Can you work these out from the model? Positions are in its coordinate system, mm. Face numbers are marked on the shaded views. A direction names the side the tool comes from. Round coordinates to 2 decimals unless told otherwise and drop trailing zeros. Order: outer loops, then holes, each group sorted by start corner. A loop starts at its lowest first (then second) coordinate and runs counter-clockwise, first axis right, second up. Notation, with made-up numbers: (86.5, 86.5) - (97.5, 86.5) arc R26 ccw to (97.5, 117.5) - close; hole circle Ø4 at (-9.5, -39). An arc over 180 degrees is marked (long way). Write item = value, one per line.
from build123d import *

# Parameters (mm, degrees)
ESQUISSE1_W             = 7.9
ESQUISSE1_H             = 8.25
BOSS_EXTRU_1_DEPTH      = 1.184
ENL_V_MAT_EXTRU_1_REACH = 15.462
BOSS_EXTRU_2_DEPTH      = 1.184
ENL_V_MAT_EXTRU_2_REACH = 15.462
ESQUISSE8_R             = 7.2925
BOSS_EXTRU_3_DEPTH      = 0.296
ESQUISSE9_R             = 6.10875
BOSS_EXTRU_4_DEPTH      = 0.74
BOSS_EXTRU_4_DRAFT      = -17.000658211
ESQUISSE10_R            = 6.335
BOSS_EXTRU_5_DEPTH      = 0.444
D_POUILLE1_ANGLE        = 44.999999999
PER_AGE1_D              = 8.376
CHANFREIN1_SIZE         = 0.812
CONG_1_R                = 0.825


with BuildPart() as part:
    # Esquisse1 → Révolution1 (revolve)
    with BuildSketch(Plane.XY, mode=Mode.PRIVATE) as r_volution1_sk:
        with Locations((5.43, 4.125)):
            Rectangle(ESQUISSE1_W, ESQUISSE1_H)
    revolve(r_volution1_sk.sketch.rotate(Axis((1.48, 0, 0), (1, 0, 0)), 270), axis=Axis((1.48, 0, 0), (1, 0, 0)))

    # Esquisse2 → Boss.-Extru.1 (add)
    with BuildSketch(Plane(origin=(9.38, 0, 0), x_dir=(0, 0, -1), z_dir=(1, 0, 0))):
        with BuildLine():
            Line((-5.652324212, -1.184), (-7.755, -1.184))
            Line((-7.755, -1.184), (-7.755, 1.184))
            Line((-7.755, 1.184), (-5.652324212, 1.184))
            ThreePointArc((-5.652324212, 1.184), (-5.775, 0), (-5.652324212, -1.184))
        make_face()
    extrude(amount=BOSS_EXTRU_1_DEPTH)

    # Esquisse4 → Enlèv. mat.-Extru.1 (cut, up to next)
    with BuildSketch(Plane(origin=(8.195, 0, 0), x_dir=(0, -1, 0), z_dir=(-1, 0, 0)), mode=Mode.PRIVATE) as enl_v_mat_extru_1_sk1:
        with BuildLine():
            Line((-2.814689148, 7.755), (2.814689148, 7.755))
            ThreePointArc((2.814689148, 7.755), (0, 8.25), (-2.814689148, 7.755))
        make_face()
    enl_v_mat_extru_1_tool1 = extrude(enl_v_mat_extru_1_sk1.sketch, amount=-ENL_V_MAT_EXTRU_1_REACH, mode=Mode.PRIVATE) & part.part
    add(enl_v_mat_extru_1_tool1.solids().sort_by_distance((8.195, 0, 7.953518))[0], mode=Mode.SUBTRACT)

    # Esquisse5 → Boss.-Extru.2 (add)
    with BuildSketch(Plane(origin=(9.38, 0, 0), x_dir=(0, 0, -1), z_dir=(1, 0, 0))):
        with BuildLine():
            Line((7.755, 1.184), (7.755, -1.184))
            Line((7.755, -1.184), (5.652324212, -1.184))
            ThreePointArc((5.652324212, -1.184), (5.775, 0), (5.652324212, 1.184))
            Line((5.652324212, 1.184), (7.755, 1.184))
        make_face()
    extrude(amount=BOSS_EXTRU_2_DEPTH)

    # Esquisse7 → Enlèv. mat.-Extru.2 (cut, up to next)
    with BuildSketch(Plane(origin=(8.195, 0, 0), x_dir=(0, -1, 0), z_dir=(-1, 0, 0)), mode=Mode.PRIVATE) as enl_v_mat_extru_2_sk1:
        with BuildLine():
            Line((2.814689148, -7.755), (-2.814689148, -7.755))
            ThreePointArc((-2.814689148, -7.755), (0, -8.25), (2.814689148, -7.755))
        make_face()
    enl_v_mat_extru_2_tool1 = extrude(enl_v_mat_extru_2_sk1.sketch, amount=-ENL_V_MAT_EXTRU_2_REACH, mode=Mode.PRIVATE) & part.part
    add(enl_v_mat_extru_2_tool1.solids().sort_by_distance((8.195, 0, -7.953518))[0], mode=Mode.SUBTRACT)

    # Esquisse8 → Boss.-Extru.3 (add)
    with BuildSketch(Plane.ZY.offset(-1.48)):
        with Locations(Location((0, 0, 0), (0, 0, 180))):
            Circle(ESQUISSE8_R)
    extrude(amount=BOSS_EXTRU_3_DEPTH)


with BuildPart() as boss_extru_4_tool:
    # Esquisse9 → Boss.-Extru.4 (with draft: the straight prism first)
    with BuildSketch(Plane.ZY.offset(-1.184)):
        Circle(ESQUISSE9_R)
    extrude(amount=BOSS_EXTRU_4_DEPTH)
    # Boss.-Extru.4: the draft: its side faces are tilted about the plane it starts from
    boss_extru_4_sides = [boss_extru_4_tool.faces().sort_by_distance(p)[0] for p in [
        (0.814, 0, -6.10875),
    ]]
    draft(boss_extru_4_sides, Plane.ZY.offset(-1.184), BOSS_EXTRU_4_DRAFT)


with BuildPart() as part_1:
    add(part.part)

    # Boss.-Extru.4: add boss_extru_4_tool
    add(boss_extru_4_tool.part)

    # Esquisse10 → Boss.-Extru.5 (add)
    with BuildSketch(Plane.ZY.offset(-0.444)):
        with Locations(Location((0, 0, 0), (0, 0, 180))):
            Circle(ESQUISSE10_R)
    extrude(amount=BOSS_EXTRU_5_DEPTH)

    # Dépouille1
    d_pouille1_faces = [part_1.faces().sort_by_distance(p)[0] for p in [
        (9.972, 0, 5.775),
        (9.972, 0, -5.775),
    ]]
    draft(d_pouille1_faces, Plane(origin=(9.38, 0, 0), x_dir=(0, 0, 1), z_dir=(1, 0, 0)), D_POUILLE1_ANGLE)

    # Perçage1 (through all)
    with Locations(Plane(origin=(9.38, 0, 0), x_dir=(0, 0, -1), z_dir=(1, 0, 0))):
        with Locations((0, 0)):
            Hole(PER_AGE1_D / 2)

    # Chanfrein1
    chanfrein1_edges = [part_1.edges().sort_by_distance(p)[0] for p in [
        (9.38, 0, -4.188),
        (0, 0, -4.188),
    ]]
    chamfer(chanfrein1_edges, length=CHANFREIN1_SIZE)

    # Congé1
    cong_1_edges = [part_1.edges().sort_by_distance(p)[0] for p in [
        (1.48, 0, 8.25),
    ]]
    fillet(cong_1_edges, radius=CONG_1_R)


solid = part_1.part
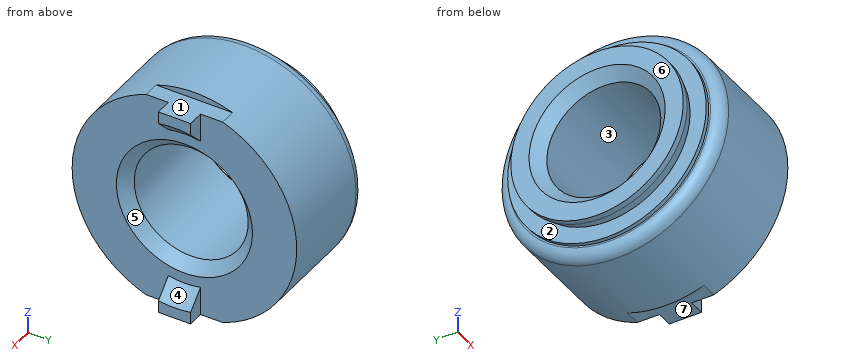
(1) Will these pins go through, and if not, where does the flat tip stop? P1, Ø0.6, axis at x = 10, z = 6.5, coming from the -Y side; P2, Ø0.9, axis at x = 9.5, z = -7, coming from the -Y side; P3, Ø4, axis at y = 1, z = 0, coming from the -X side; P4, Ø5, axis at x = 6.5, y = -6.5, coming from the +Z side.
Computed:
P1 = -1.18
P2 = -4.99
P3 = through
P4 = 7.22
(2) If I drill on line 1 (Y direction, x = 3.75, z = 0); line 2 (X direction, y = -2.5, z = 6.5); line 3 (Y direction, x = 7.75, z = -3.5), over which ranges is the centre line in solid material (lowest first)? Write a range as from..to.
Computed:
line_1 = -8.25..-4.19, 4.19..8.25
line_2 = 1.18..9.38
line_3 = -7.47..-2.3, 2.3..7.47
(3) If we section it at C-C (x = 4.5): Write out the boundary of the cut face in (y, z).
Computed:
outline = circle Ø16.5 at (0, 0); hole circle Ø8.38 at (0, 0)
(4) On a 3-axis mill with a long thin cutter (end or side, diameter ignored), from which of +Z, -Z, +X, -X, +Y, -Y can I reach the whole of each face in a straight line? I mean the marked faces 1, 2 and 3. Say none if no direction works.
Computed:
face_1 = +Z, +X, +Y, -Y
face_2 = none
face_3 = +X, -X
(5) Thinking about a two-plate mould opening in Z: for the marked faces 4, 5, 6 and 7, which applies, +Z half, -Z half, draft (parallel to the pull), parting line (faces both ways), or undercut?
Computed:
face_4 = undercut
face_5 = undercut
face_6 = draft
face_7 = -Z half
